```python
from build123d import *

# Parameters (mm, degrees)
F1_DEPTH = 25
F2_R     = 12.5
F3_DEPTH = 10


with BuildPart() as f1:
    # F0 (on Top) → F1 (new body)
    with BuildSketch(Plane.XY):
        with BuildLine():
            Line((17.320508, 30), (-17.320508, 30))
            ThreePointArc((-17.320508, 30), (-34.641016, 20), (-34.641016, 0))
            Line((-34.641016, 0), (-17.320508, -30))
            ThreePointArc((-17.320508, -30), (0, -40), (17.320508, -30))
            Line((17.320508, -30), (34.641016, 0))
            ThreePointArc((34.641016, 0), (34.641016, 20), (17.320508, 30))
        make_face()
    extrude(amount=F1_DEPTH)

    # F2 (on face) → F3 (cut)
    with BuildSketch(Plane.XY.offset(25)):
        with Locations((-17.320508, 10)):
            Circle(F2_R)
        with Locations((0, -20)):
            Circle(F2_R)
        with Locations((17.320508, 10)):
            Circle(F2_R)
    extrude(amount=-F3_DEPTH, mode=Mode.SUBTRACT)


solid = f1.part
```
Here's how the part is built. I have some questions about the finished solid (model axes, mm). A direction names the side the tool comes from. Give positions to 0.01 mm unless a question says otherwise; leave off trailing zeros. Order: outer loops, then holes, each group sorted by start corner. A loop starts at its lowest first (then second) coordinate and runs counter-clockwise, first axis right, second up. Notation, with made-up numbers: (42, 46.5) -> (68, 46.5) arc R9 cw to (68, 57.5) -> close; hole circle Ø4 at (-29.75, -38.5). An arc over 180 degrees is marked (long way). Use CSV: the item, a comma, the result in double quotes. Start each with the question number.
Item 1: Suppose I cut it at B-B (z = 23). List the corners of the cut face in (x, y) for me.
Item 2: On a 3-axis mill with a long thin cutter (end or side, diameter ignored), from which of +Z, -Z, +X, -X, +Y, -Y can I reach the whole of each face in a straight line? I mean faces 1 (the cylindrical face through (-2.71, -32.203, 20.07)), 2 (the flat face through (25.86, -15.21, 12.32)). Say none if no direction works.
Item 3: If I drill on probe 1 along Y at (x, z) = (-6.5, 23.75); probe 2 along X at (y, z) = (16, 16.25); probe 3 along Y at (x, z) = (0, 22.5), over which ranges is the centre line in solid material (lowest first)? Write a range as [from, to].
Item 4: Suppose I cut it at D-D (z = 10.25). List the corners of the cut face in (x, y) for me.
Item 5: I'm going to push flat-ended pins straight in: P1, Ø22.5, axis at x = 0, y = -20, coming from the -Z side; P2, Ø5, axis at x = -26, y = 6.5, coming from the +Z side; P3, Ø1, axis at x = -4, z = 6, coming from the -Y side; P4, Ø1.5, axis at x = -21, z = 15, coming from the -Y side. Where does each tip first touch, or does it pass through?
Item 6: Suppose I cut it at A-A (x = 0). List the corners of the cut face in (y, z) for me.
Item 7: Suppose I cut it at C-C (y = -20). List the corners of the cut face in (x, z) for me, and give its area (3 significant figures).
Answer block:
1,outline,"(-34.64, 0) -> (-17.32, -30) arc R20 ccw to (17.32, -30) -> (34.64, 0) arc R20 ccw to (17.32, 30) -> (-17.32, 30) arc R20 ccw to start; hole circle Ø25 at (-17.32, 10); hole circle Ø25 at (0, -20); hole circle Ø25 at (17.32, 10)"
2,face 1,"+Z"
2,face 2,"+Z, -Z, +X, -Y"
3,probe 1,"y = [-38.91, -30.68], [-9.32, 3.74], [16.26, 30]"
3,probe 2,"x = [-36.4, -28.29], [-6.35, 6.35], [28.29, 36.4]"
3,probe 3,"y = [-40, -32.5], [-7.5, 30]"
4,outline,"(-34.64, 0) -> (-17.32, -30) arc R20 ccw to (17.32, -30) -> (34.64, 0) arc R20 ccw to (17.32, 30) -> (-17.32, 30) arc R20 ccw to start"
5,P1,"stops at z = 0"
5,P2,"stops at z = 15"
5,P3,"stops at y = -39.69"
5,P4,"stops at y = -24.93"
6,outline,"(-40, 0) -> (30, 0) -> (30, 25) -> (-7.5, 25) -> (-7.5, 15) -> (-32.5, 15) -> (-32.5, 25) -> (-40, 25) -> close"
7,outline,"(-23.09, 0) -> (23.09, 0) -> (23.09, 25) -> (12.5, 25) -> (12.5, 15) -> (-12.5, 15) -> (-12.5, 25) -> (-23.09, 25) -> close"
7,area,"905 mm^2"
